Autodesk Inventor part; units mm, degrees
ref_plane "YZ Plane" through (0, 0, 0) normal (1, 0, 0) x (0, 1, 0)
ref_plane "XZ Plane" through (0, 0, 0) normal (0, 1, 0) x (-1, 0, 0)
ref_plane "XY Plane" through (0, 0, 0) normal (0, 0, 1) x (1, 0, 0)
sketch "Sketch2" plane through (0, 0, 0) normal (0, 0, 1) x (1, 0, 0)
  line L0 (0, -25.4) -> (0, 25.4) construction
  line L1 (17.4625, -25.4) -> (17.4625, 25.4)
  line L2 (-17.4625, 25.4) -> (-17.4625, -25.4)
  circle A0 centre (0, -25.4) radius 14.2875 construction
  circle A1 centre (0, 25.4) radius 14.2875 construction
  line L3 (-14.2875, -15.3598) -> (-14.2875, 15.218)
  line L4 (7.2043, -9.4928) -> (-14.2875, 15.218)
  line L5 (14.2875, -15.218) -> (-7.2043, 9.4928)
  line L6 (14.2875, -15.218) -> (14.2875, 15.3598)
  arc A2 (-17.4625, -25.4) -> (17.4625, -25.4) centre (0, -25.4) ccw
  arc A3 (7.2043, -9.4928) -> (-14.2875, -15.3598) centre (0, -25.4) ccw
  arc A4 (17.4625, 25.4) -> (-17.4625, 25.4) centre (0, 25.4) ccw
  arc A5 (-7.2043, 9.4928) -> (14.2875, 15.3598) centre (0, 25.4) ccw
  point P0 (0, 0)
  dimension "d3" = 28.575
  dimension "d4" = 50.8
  dimension "d15" = 1.5875
  dimension "d16" = 17.4625
  dimension "d18" = 3.175
extrude "Extrusion1" add sketch "Sketch2" along normal mid plane 6.35
sketch "Sketch3" plane through (0, 0, 3.175) normal (0, 0, 1) x (1, 0, 0)
  arc A0 (-17.4625, -25.4) -> (17.4625, -25.4) centre (0, -25.4) ccw construction
  arc A1 (17.4625, 25.4) -> (-17.4625, 25.4) centre (0, 25.4) ccw construction
  point P0 (0, 0)
  point P1 (0, 25.4)
hole "Hole1" at (0, -25.4, 3.175) at (0, 25.4, 3.175) direction (0, 0, -1) diameter 27.94 end through all
fillet "Fillet1" radius 1.5875 6 edges at (14.2875, -15.218, 0) (7.2043, -9.4928, 0) (14.2875, 15.3598, 0) (-7.2043, 9.4928, 0) (-14.2875, -15.3598, 0) (-14.2875, 15.218, 0)
properties part number "BRACE,SHAFT,ELEVATOR" material "Aluminum 7075"
Work out the finished part from the listing and answer in its coordinate system (mm). A direction names the side the tool comes from. Round coordinates to 2 decimals unless told otherwise and drop trailing zeros. Loops run counter-clockwise (first coordinate to the right, second up) from the corner with the lowest first, then second, coordinate; pieces in that order, holes last. Notation, with made-up numbers: M 61.5,-0.5 L 113.5,-0.5 A15 cw 113.5,23.5 Z; hole C -16.5,-22 d11. An arc over 180 degrees is marked long. One line per question, with ' | ' between items.
Q1. Find section A-A, the plane y = -20.5. Give the vertices of the cut face in (x, z) (1 decimal), then the cut area to 3 significant figures.
Conclusion:
outline: M -17.5,-3.2 L -13.1,-3.2 L -13.1,3.2 L -17.5,3.2 Z; M 13.1,-3.2 L 17.5,-3.2 L 17.5,3.2 L 13.1,3.2 Z | area: 55.6 mm2
Q2. Find section C-C, the plane x = 10.5. Give the vertices of the cut face in (y, z) (3 decimals).
Conclusion:
outline: M -39.353,-3.175 L -34.615,-3.175 L -34.615,3.175 L -39.353,3.175 Z; M -16.185,-3.175 L -10.863,-3.175 L -10.863,3.175 L -16.185,3.175 Z; M 11.447,-3.175 L 16.185,-3.175 L 16.185,3.175 L 11.447,3.175 Z; M 34.615,-3.175 L 39.353,-3.175 L 39.353,3.175 L 34.615,3.175 Z
Q3. The mould has two halves that part along X. Classify faces 1 (the flat face through (17.462, 0, 0)), 2 (the flat face through (-0.2, 0.6, -3.175)), 3 (the flat face through (-14.288, 0, 0)): +X half, -X half, draft (parallel to the pull), parting line (faces both ways), or undercut.
Conclusion:
face 1: +X half | face 2: draft | face 3: undercut
Q4. Find section B-B, the plane x = 0. Give the vertices of the cut face in (y, z) (1 decimal), then the cut area to 3 significant figures.
Conclusion:
outline: M -42.9,-3.2 L -39.4,-3.2 L -39.4,3.2 L -42.9,3.2 Z; M -11.4,-3.2 L -7.9,-3.2 L -7.9,3.2 L -11.4,3.2 Z; M -1.2,-3.2 L 1.2,-3.2 L 1.2,3.2 L -1.2,3.2 Z; M 7.9,-3.2 L 11.4,-3.2 L 11.4,3.2 L 7.9,3.2 Z; M 39.4,-3.2 L 42.9,-3.2 L 42.9,3.2 L 39.4,3.2 Z | area: 104 mm2
Q5. Consider line 1 along Y through (x, z) = (12.5, 2.75); line 2 along Y through (x, z) = (3.5, -1.25); line 3 along X through (y, z) = (25.4, -0.5). Determine where each line is inside the solid, lowest interval first. Write a range as from..to.
Conclusion:
line 1: y = -37.59..-31.64, -19.16..-12.55, 12.78..19.16, 31.64..37.59 | line 2: y = -42.51..-38.92, -11.88..-7.76, -5.23..-2.81, 8.29..11.88, 38.92..42.51 | line 3: x = -17.46..-13.97, 13.97..17.46
Q6. A tool of negligible diameter and unlimited length cuts with its end or side. For faces 4 (the flat face through (14.288, 0, 0)), 5 (the cylindrical face through (0.38, -42.86, -0.04)), from which of +Z, -Z, +X, -X, +Y, -Y can it reach the whole face along a straight path? Write none if from no direction.
Conclusion:
face 4: +Z, -Z | face 5: +Z, -Z, -Y
Q7. Each of these flat-tipped pins is pushed along its axis until it touches: pin 1 Ø6 at (x, y) = (9, -27.5) entering from +Z (3 decimals); pin 2 Ø2 at (x, z) = (8, 0.5) entering from -Y. Where does it stop, or does it pass through?
Conclusion:
pin 1: passes through | pin 2: stops at y = -41.4
Q8. Find section D-D, the plane z = 0.5. Give the vertices of the cut face in (x, y) (1 decimal).
Conclusion:
outline: M -17.5,-25.4 A17.5 ccw 17.5,-25.4 L 17.5,25.4 A17.5 ccw -17.5,25.4 Z; hole M -14.3,-11.2 A1.6 ccw -11.6,-12.4 A17.5 cw 2.3,-8.1 A1.6 ccw 3.7,-5.5 L -11.5,12 A1.6 ccw -14.3,11 Z; hole C 0,-25.4 d27.9; hole C 0,25.4 d27.9; hole M -3.7,5.5 L 11.5,-12 A1.6 ccw 14.3,-11 L 14.3,11.2 A1.6 ccw 11.6,12.4 A17.5 cw -2.3,8.1 A1.6 ccw Z
